Source: three-view drawing plus pictorial views. Frame: mm from the lowest corner of the part. Round coordinates to 2 decimals unless told otherwise and drop trailing zeros. Loops run counter-clockwise (first coordinate to the right, second up) from the corner with the lowest first, then second, coordinate; pieces in that order, holes last. Notation, with made-up numbers: M 55,75.25 L 108,75.25 A30 cw 108,100.25 Z; hole C 43.25,-11.75 d8. An arc over 180 degrees is marked long. Answer as a JSON object with one key per item and string values.
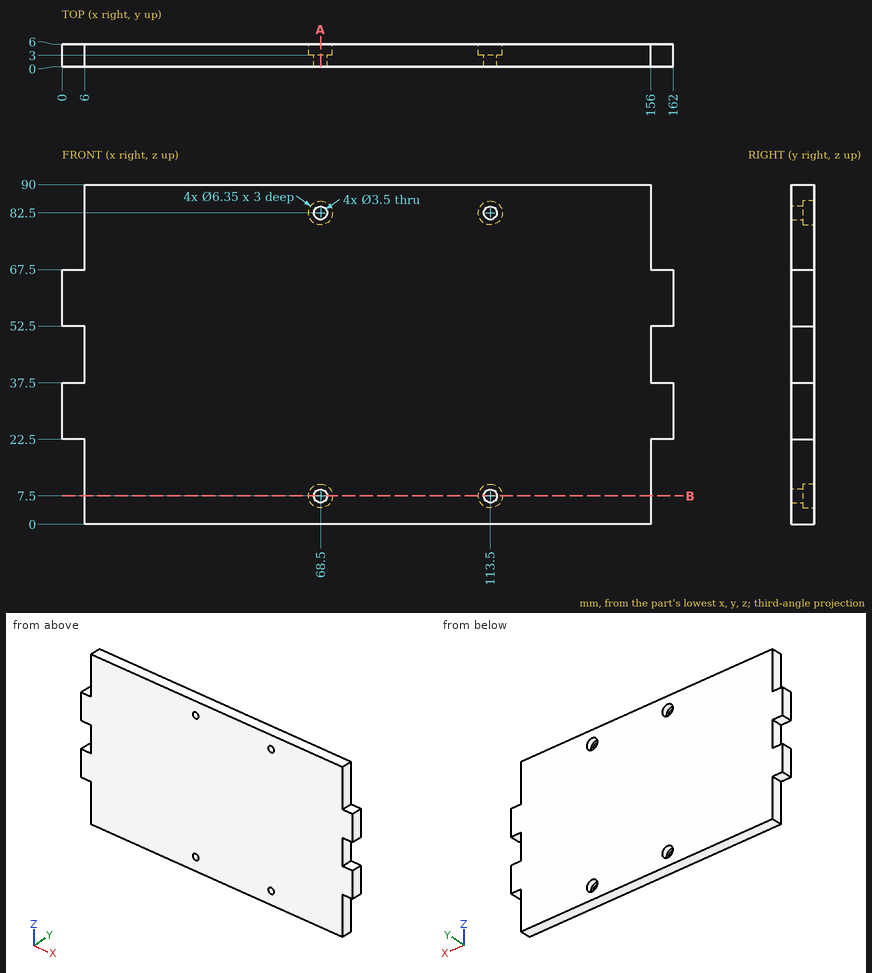
1) Cut plane A-A on x = 68.5. Return the cut outline in (y, z) (3 decimals), and give its area (3 significant figures).
Geometry results:
{"outline": "M 0,0 L 6,0 L 6,4.325 L 3,4.325 L 3,5.75 L 0,5.75 Z; M 0,9.25 L 3,9.25 L 3,10.675 L 6,10.675 L 6,79.325 L 3,79.325 L 3,80.75 L 0,80.75 Z; M 0,84.25 L 3,84.25 L 3,85.675 L 6,85.675 L 6,90 L 0,90 Z", "area": "481 mm2"}
2) First-contact query: pin 1 (1.8 mm diameter, centred on x = 3.5, y = 2.5, fed in from -Z); pin 2 (4 mm diameter, centred on x = 113.5, z = 82.5, fed in from +Y); pin 3 (1 mm diameter, centred on y = 4, z = 44, fed in from -X). Flat tips, straight axial feed; report the tip coordinate or a pass-through.
Geometry results:
{"pin 1": "z = 22.5", "pin 2": "y = 3", "pin 3": "x = 6"}
3) Cut plane B-B on z = 7.5. Return the cut outline in (x, y) (3 decimals), and give its area (3 significant figures).
Geometry results:
{"outline": "M 6,0 L 66.75,0 L 66.75,3 L 65.325,3 L 65.325,6 L 6,6 Z; M 70.25,0 L 111.75,0 L 111.75,3 L 110.325,3 L 110.325,6 L 71.675,6 L 71.675,3 L 70.25,3 Z; M 115.25,0 L 156,0 L 156,6 L 116.675,6 L 116.675,3 L 115.25,3 Z", "area": "841 mm2"}
4) Line query: probe 1 along X at (y, z) = (5.3, 7.5) (3 decimals); probe 2 along X at (y, z) = (0.85, 82.5); probe 3 along Z at (x, y) = (68.5, 1.4). Output: solid intervals per line, ascending.
Geometry results:
{"probe 1": "6 to 65.325, 71.675 to 110.325, 116.675 to 156", "probe 2": "6 to 66.75, 70.25 to 111.75, 115.25 to 156", "probe 3": "0 to 5.75, 9.25 to 80.75, 84.25 to 90"}
